Job drawing, mm, ordinate dimensions from the low corner. One solid piece. A direction names the side the tool comes from. Coordinates: 2 decimals unless noted, no trailing zeros. Write each loop counter-clockwise with the first axis right and the second up, starting at its lowest first coordinate (ties: lowest second). Pieces come first, ordered by that corner, then holes. Notation, with made-up numbers: (-35.5, -35.5) - (21.5, -35.5) arc R15 cw to (21.5, -8.5) - close; hole circle Ø9 at (38.5, 38.5). An arc over 180 degrees is marked (long way). Put each result on its own line as item: value. Start each with the question number.
1. Which spindle directions (+Z, -Z, +X, -X, +Y, -Y) get a long thin tool onto all of the face, cutting with end or side? Do the marked faces 4 and 5. Say none if no direction does.
2. Saw through at B-B, the plane y = 5. Write the cut outline in (x, z), plus the area to 3 significant figures.
3. Saw through at C-C, the plane z = 3.25. Write the cut outline in (x, y), plus the area to 3 significant figures.
4. Saw through at A-A, the plane x = 34.5. Write the cut outline in (y, z).
5. Drill centre lines: L1, parallel to Y at x = 5.5, z = 3.5; L2, parallel to X at y = 5.75, z = 2.75; L3, parallel to X at y = 5.25, z = 5.25. Where is each one in solid material? Low to high. Write a range as from..to.
6. Drop flat-ended pins along their axis: P1, Ø6, axis at x = 34.5, y = 5, coming from the -Z side; P2, Ø1.6, axis at x = 35, y = 4.5, coming from the -Z side. Give the stop position or say it passes through.
7. Pull direction X, two halves, no side cores. Call the marked faces 1, 2 and 3: released by +X, released by -X, zero draft, split by the parting line, or undercut.
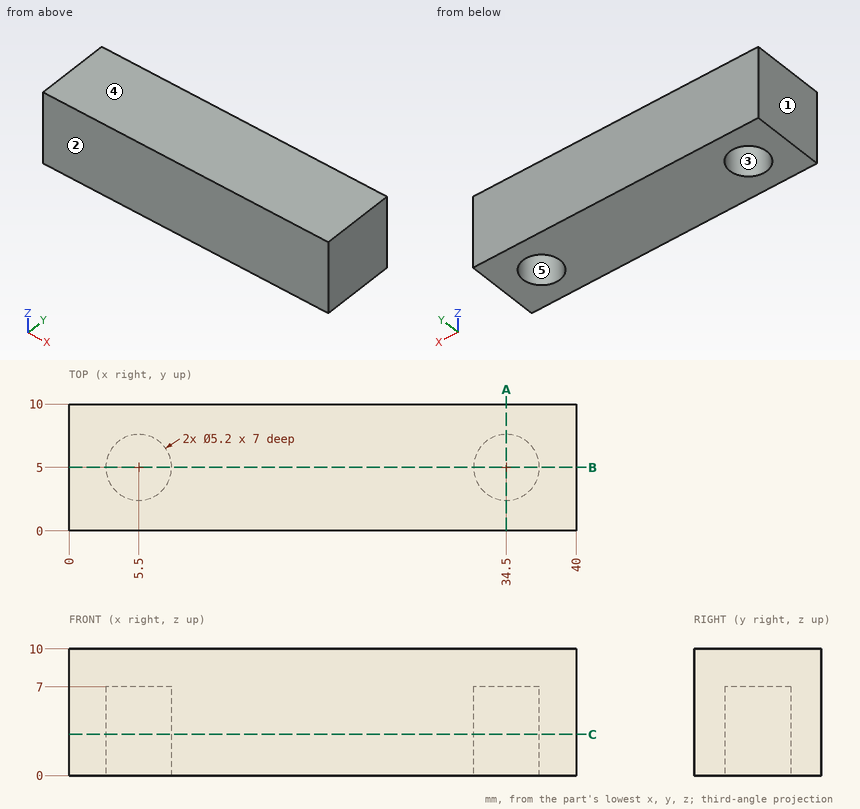
Final values:
1. face 4: +Z, +X, -X, +Y, -Y
1. face 5: -Z
2. outline: (0, 0) - (2.9, 0) - (2.9, 7) - (8.1, 7) - (8.1, 0) - (31.9, 0) - (31.9, 7) - (37.1, 7) - (37.1, 0) - (40, 0) - (40, 10) - (0, 10) - close
2. area: 327 mm²
3. outline: (0, 0) - (40, 0) - (40, 10) - (0, 10) - close; hole circle Ø5.2 at (5.5, 5); hole circle Ø5.2 at (34.5, 5)
3. area: 358 mm²
4. outline: (0, 0) - (2.4, 0) - (2.4, 7) - (7.6, 7) - (7.6, 0) - (10, 0) - (10, 10) - (0, 10) - close
5. L1: y = 0..2.4, 7.6..10
5. L2: x = 0..3.01, 7.99..32.01, 36.99..40
5. L3: x = 0..2.91, 8.09..31.91, 37.09..40
6. P1: stops at z = 0
6. P2: stops at z = 7
7. face 1: released by -X
7. face 2: zero draft
7. face 3: undercut
